Could you check a few things on this model? Use its own coordinates, in mm. A direction names the side the tool comes from. Coordinates: 2 decimals unless noted, no trailing zeros. Order: outer loops, then holes, each group sorted by start corner. A loop starts at its lowest first (then second) coordinate and runs counter-clockwise, first axis right, second up. Notation, with made-up numbers: (-10.75, 72) -> (21.25, 72) arc R16 cw to (21.25, 78) -> close; hole circle Ø8 at (11.25, -25.75). An arc over 180 degrees is marked (long way). Use a Markdown table: item, result. Add a question column.
1) If we section it at C-C (y = 45.5): Write out the boundary of the cut face in (x, z), plus the area to 3 significant figures.
2) If we section it at B-B (z = 21): Write out the boundary of the cut face in (x, y).
3) If we section it at A-A (x = 80.5): Write out the boundary of the cut face in (y, z) (3 decimals), plus the area to 3 significant figures.
4) If I drill on L1, parallel to Y at x = 60, z = 27, over which ranges is the centre line in solid material (lowest first)? Write a range as [from, to].
5) Which directions (+Z, -Z, +X, -X, +Y, -Y) give clear straight access to the entire face, cutting with the end or side of a thin tool? Please do faces 1 (the cylindrical face through (45.07, -2.84, 0.95)), 2 (the flat face through (57.15, 41, 19)).
6) Thinking about a two-plate mould opening in Y: for faces 3 (the flat face through (73, 34.351, 19)), 4 (the flat face through (44, -3.749, 19)), 5 (the flat face through (44, 41, 38.1)), which applies, +Y half, -Y half, draft (parallel to the pull), parting line (faces both ways), or undercut?
Autodesk Inventor part; units mm, degrees
ref_plane "YZ Plane" through (0, 0, 0) normal (1, 0, 0) x (0, 1, 0)
ref_plane "XZ Plane" through (0, 0, 0) normal (0, 1, 0) x (-1, 0, 0)
ref_plane "XY Plane" through (0, 0, 0) normal (0, 0, 1) x (1, 0, 0)
sketch "Sketch1" plane through (0, 0, 0) normal (1, 0, 0) x (0, 1, 0)
  line L0 (-3.7488, 0) -> (85.1512, 0)
  line L1 (85.1512, 0) -> (85.1512, 38.1)
  line L2 (85.1512, 38.1) -> (-3.7488, 38.1)
  line L3 (-3.7488, 38.1) -> (-3.7488, 0)
  point P0 (0, 0)
  dimension "d0" = 88.9
  dimension "d1" = 38.1
extrude "Extrusion1" add sketch "Sketch1" along normal blind 88.9
fillet "Fillet1" radius 3.175 4 edges at (44.45, 85.1512, 38.1) (44.45, 85.1512, 0) (44.45, -3.7488, 0) (44.45, -3.7488, 38.1)
sketch "Sketch2" plane through (88.9, 0, 0) normal (1, 0, 0) x (0, 0, -1)
  line L0 (-34.925, -3.7488) -> (-3.175, -3.7488)
  line L1 (0, -0.5738) -> (0, 81.9762)
  line L2 (-3.175, 85.1512) -> (-34.925, 85.1512)
  line L3 (-38.1, 81.9762) -> (-38.1, -0.5738)
  line L4 (-38.1, 47.0512) -> (0, 47.0512)
  line L5 (0, 47.0512) -> (0, 34.3512)
  line L6 (0, 34.3512) -> (-38.1, 34.3512)
  line L7 (-38.1, 34.3512) -> (-38.1, 47.0512)
  point P0 (0, 0)
  dimension "d5" = 38.1
  dimension "d6" = 38.1
extrude "Extrusion2" cut sketch "Sketch2" against normal blind 31.75
properties part number "2x4x3.5" material "Ash"
Answer sheet:
| question | item | result |
|---|---|---|
| 1 | outline | (0, 0) -> (57.15, 0) -> (57.15, 38.1) -> (0, 38.1) -> close |
| 1 | area | 2,180 mm2 |
| 2 | outline | (0, -3.75) -> (88.9, -3.75) -> (88.9, 34.35) -> (57.15, 34.35) -> (57.15, 47.05) -> (88.9, 47.05) -> (88.9, 85.15) -> (0, 85.15) -> close |
| 3 | outline | (-3.749, 3.175) arc R3.175 ccw to (-0.574, 0) -> (34.351, 0) -> (34.351, 38.1) -> (-0.574, 38.1) arc R3.175 ccw to (-3.749, 34.925) -> close; (47.051, 0) -> (81.976, 0) arc R3.175 ccw to (85.151, 3.175) -> (85.151, 34.925) arc R3.175 ccw to (81.976, 38.1) -> (47.051, 38.1) -> close |
| 3 | area | 2,890 mm2 |
| 4 | L1 | [-3.75, 34.35], [47.05, 85.15] |
| 5 | face 1 | -Z, +X, -X, -Y |
| 5 | face 2 | +Z, -Z, +X |
| 6 | face 3 | undercut |
| 6 | face 4 | -Y half |
| 6 | face 5 | draft |
